The model under review builds one solid part; all positions refer to its coordinate system, in mm. A direction names the side the tool comes from. Coordinates: 2 decimals unless noted, no trailing zeros. Write each loop counter-clockwise with the first axis right and the second up, starting at its lowest first coordinate (ties: lowest second). Pieces come first, ordered by that corner, then holes. Notation, with made-up numbers: (-27, -21) - (-8, -21) arc R16 ccw to (-8, 7) - close; hole circle Ø9 at (67.25, 61). An arc over 180 degrees is marked (long way). Put each result on its own line as item: value.
from build123d import *

# Parameters (mm, degrees)
F1_DEPTH    = 10
F2_SIZE     = 1.2
F3_R        = 0.5
F5_W        = 9.8
F5_H        = 7.9
F6_DEPTH    = 5
F8_DEPTH    = 2.2
F9_T1_DEPTH = 9.6433659759
F10_R       = 1


# Not quite as in the source:
# - a fillet or chamfer that OpenCascade refuses, or shapes differently, is made with other operations: its cross-section is extruded or revolved along the edge and cut away or added


with BuildPart() as f1:
    # F0 (on Front) → F1 (new body)
    with BuildSketch(Plane.XZ):
        Polygon((-3.45, 2.8), (-3.45, 0), (3.45, 0), (3.45, 2.8), (2.925, 2.8), (2.925, 4.4), (-2.925, 4.4), (-2.925, 2.8), align=None)
    extrude(amount=F1_DEPTH)

    # F2
    f2_edges = [f1.edges().sort_by_distance(p)[0] for p in [
        (3.45, -10, 1.4),
        (-3.45, -10, 1.4),
    ]]
    chamfer(f2_edges, length=F2_SIZE)

    # F3
    f3_edges = [f1.edges().sort_by_distance(p)[0] for p in [
        (-3.45, -4.4, 0),
        (3.45, -4.4, 0),
    ]]
    fillet(f3_edges, radius=F3_R)

    # F5 (on Front) → F6 (join)
    with BuildSketch(Plane.XZ):
        with Locations((0, 2.92)):
            Rectangle(F5_W, F5_H)
    extrude(amount=-F6_DEPTH)

    # F7 (on offset) → F8 (cut)
    with BuildSketch(Plane.XY.offset(4.4)):
        Polygon((-1.5, 0), (-1.5, -9), (-0.5, -9), (-0.5, 5), (-1.5, 5), align=None)
        Polygon((1.5, 5), (0.5, 5), (0.5, -9), (1.5, -9), (1.5, 0), align=None)
    extrude(amount=-F8_DEPTH, mode=Mode.SUBTRACT)

    # F9: chamfer of 1 on 1 edges, made by hand

    # F9_s2 → F9_t1 (cut)
    with BuildSketch(Plane.YZ.offset(-4.821682988)):
        Polygon((-9, 0), (-10, 1), (-10, 0), align=None)
    extrude(amount=F9_T1_DEPTH, mode=Mode.SUBTRACT)

    # F10
    f10_edges = [f1.edges().sort_by_distance(p)[0] for p in [
        (4.9, 2.5, 6.87),
        (4.9, 2.5, -1.03),
        (-4.9, 2.5, -1.03),
        (-4.9, 2.5, 6.87),
    ]]
    fillet(f10_edges, radius=F10_R)


solid = f1.part
1. For pin 1 Ø4 at (x, y) = (0.5, -7) entering from -Z; pin 2 Ø1.8 at (y, z) = (-3, 4) entering from +X (3 decimals); pin 3 Ø0.8 at (x, y) = (-1, -4) entering from +Z; pin 4 Ø5 at (x, y) = (0, -1.5) entering from +Z, all flat-tipped, find the tip position at first contact; note any pin that passes through.
Determined:
pin 1: stops at z = 0
pin 2: stops at x = 2.925
pin 3: stops at z = 2.2
pin 4: stops at z = 6.87
2. Consider section B-B on y = 2.75. State the section outline as (x, z) points.
Determined:
outline: (-4.9, -0.03) arc R1 ccw to (-3.9, -1.03) - (3.9, -1.03) arc R1 ccw to (4.9, -0.03) - (4.9, 5.87) arc R1 ccw to (3.9, 6.87) - (-3.9, 6.87) arc R1 ccw to (-4.9, 5.87) - close; hole (-1.5, 2.2) - (-0.5, 2.2) - (-0.5, 4.4) - (-1.5, 4.4) - close; hole (0.5, 2.2) - (1.5, 2.2) - (1.5, 4.4) - (0.5, 4.4) - close
3. The part is to be moulded in two halves that separate along X. For faces 1 (the flat face through (0, -10, 3)), 2 (the flat face through (-1.5, -2, 3)), 3 (the flat face through (3.45, -4, 2)), say which applies: +X half, -X half, draft (parallel to the pull), parting line (faces both ways), or undercut.
Determined:
face 1: draft
face 2: undercut
face 3: +X half
4. Consider section D-D on x = 2.5. State the section outline as (y, z) points.
Determined:
outline: (-9.75, 0.75) - (-9, 0) - (0, 0) - (0, -1.03) - (5, -1.03) - (5, 6.87) - (0, 6.87) - (0, 4.4) - (-9.75, 4.4) - close
5. Machinability: for faces 4 (the flat face through (0, -5, 4.4)), 5 (the flat face through (2.925, -5, 4)), 6 (the flat face through (0, -4, 0)), 7 (the flat face through (-2.925, -5, 4)), 8 (the flat face through (1, -9, 3)), which of the approach directions +Z, -Z, +X, -X, +Y, -Y give a long, thin tool a straight path to every point of the face, cutting with its end or side? Answer none if there is none.
Determined:
face 4: +Z, +X, -X, -Y
face 5: +Z, +X, -Y
face 6: -Z, +X, -X, -Y
face 7: +Z, -X, -Y
face 8: +Z, +Y
6. To check wall thickness, follow probe 1 along X at (y, z) = (0.5, 3.5); probe 2 along X at (y, z) = (-3, 4.25) (3 decimals); probe 3 along Z at (x, y) = (-0.75, 4.75). State the ranges of each line that lie inside material, in increasing order.
Determined:
probe 1: x = -4.9 to -1.5, -0.5 to 0.5, 1.5 to 4.9
probe 2: x = -2.925 to -1.5, -0.5 to 0.5, 1.5 to 2.925
probe 3: z = -1.03 to 2.2, 4.4 to 6.87
7. Consider section C-C on z = 3.5. State the section outline as (x, y) points (3 decimals).
Determined:
outline: (-4.9, 0) - (-2.925, 0) - (-2.925, -9.325) - (-2.25, -10) - (2.25, -10) - (2.925, -9.325) - (2.925, 0) - (4.9, 0) - (4.9, 5) - (1.5, 5) - (1.5, -9) - (0.5, -9) - (0.5, 5) - (-0.5, 5) - (-0.5, -9) - (-1.5, -9) - (-1.5, 5) - (-4.9, 5) - close
8. Consider section A-A on x = 1. State the section outline as (y, z) points.
Determined:
outline: (-10, 1) - (-9, 0) - (0, 0) - (0, -1.03) - (5, -1.03) - (5, 2.2) - (-9, 2.2) - (-9, 4.4) - (-10, 4.4) - close; (0, 4.4) - (5, 4.4) - (5, 6.87) - (0, 6.87) - close
